Can you work these out from the model? Positions are in its coordinate system, mm. A direction names the side the tool comes from. Give positions to 0.01 mm unless a question says otherwise; leave off trailing zeros. Loops run counter-clockwise (first coordinate to the right, second up) from the corner with the lowest first, then second, coordinate; pieces in that order, holes last. Notation, with made-up numbers: (26, 58) - (71, 58) arc R18 ccw to (71, 93) - close; hole circle Ø9 at (-22, 18). An arc over 180 degrees is marked (long way). Answer as a JSON object with one key per item and string values.
```python
from build123d import *

# Parameters (mm, degrees)
F0_W     = 88.9
F0_H     = 88.9
F1_DEPTH = 2.54
F2_W     = 81.28
F2_H     = 81.28
F2_W_2   = 73.834833
F2_H_2   = 73.66
F3_DEPTH = 6.35
F4_R     = 1.27
F5_DEPTH = 2.541


with BuildPart() as f1:
    # F0 (on Top) → F1 (new body)
    with BuildSketch(Plane.XY):
        with Locations((44.45, 44.45)):
            Rectangle(F0_W, F0_H)
    extrude(amount=F1_DEPTH)

    # F2 (on face) → F3 (join)
    with BuildSketch(Plane.XY.offset(2.54)):
        with Locations((44.45, 44.45)):
            Rectangle(F2_W, F2_H)
        with Locations((44.362583, 44.45)):
            Rectangle(F2_W_2, F2_H_2, mode=Mode.SUBTRACT)
    extrude(amount=F3_DEPTH)

    # F4 (on face) → F5 (cut, through all)
    with BuildSketch(Plane.XY.offset(2.54)):
        with Locations((11.041525, 77.692158)):
            Circle(F4_R)
        with Locations((77.683642, 77.692158)):
            Circle(F4_R)
        with Locations((77.683642, 11.207842)):
            Circle(F4_R)
        with Locations((11.041525, 11.207842)):
            Circle(F4_R)
    extrude(amount=-F5_DEPTH, mode=Mode.SUBTRACT)


solid = f1.part
```
1) Imagine slicing it at B-B on y = 37. Write out the boundary of the cut face in (x, z), and give its area (3 significant figures).
Check sheet entries:
{"outline": "(0, 0) - (88.9, 0) - (88.9, 2.54) - (85.09, 2.54) - (85.09, 8.89) - (81.28, 8.89) - (81.28, 2.54) - (7.45, 2.54) - (7.45, 8.89) - (3.81, 8.89) - (3.81, 2.54) - (0, 2.54) - close", "area": "273 mm2"}
2) Which directions (+Z, -Z, +X, -X, +Y, -Y) give clear straight access to the entire face, cutting with the end or side of a thin tool? Please do faces 5 (the flat face through (44, 85.09, 6)), 6 (the flat face through (44, 81.28, 6)), 7 (the flat face through (3.81, 44, 6)).
Check sheet entries:
{"face 5": "+Z, +X, -X, +Y", "face 6": "+Z", "face 7": "+Z, -X, +Y, -Y"}
3) If we mould it in two halves opening along Y, with no side actions, what happens to faces 1 (the flat face through (44, 45, 2.54)), 2 (the flat face through (88.9, 44, 1)), 3 (the flat face through (44, 7.62, 6)), 4 (the flat face through (44, 88.9, 1))? For each: released by +Y, released by -Y, zero draft, split by the parting line, or undercut.
Check sheet entries:
{"face 1": "undercut", "face 2": "zero draft", "face 3": "undercut", "face 4": "released by +Y"}
4) Imagine slicing it at C-C on x = 80. Write out the boundary of the cut face in (y, z), and give its area (3 significant figures).
Check sheet entries:
{"outline": "(0, 0) - (88.9, 0) - (88.9, 2.54) - (85.09, 2.54) - (85.09, 8.89) - (81.28, 8.89) - (81.28, 2.54) - (7.62, 2.54) - (7.62, 8.89) - (3.81, 8.89) - (3.81, 2.54) - (0, 2.54) - close", "area": "274 mm2"}
5) I'm going to push flat-ended pins straight in: P1, Ø3, axis at x = 77.68, y = 11.21, coming from the +Z side; P2, Ø5, axis at x = 52, z = 6.5, coming from the +Y side; P3, Ø1.5, axis at y = 60, z = 7.5, coming from the +X side. Where does each tip first touch, or does it pass through?
Check sheet entries:
{"P1": "z = 2.54", "P2": "y = 85.09", "P3": "x = 85.09"}
6) I need wall thicknesses on L1, parallel to X at y = 66, z = 6.25; L2, parallel to Y at x = 8.5, z = 3.75; L3, parallel to Z at x = 8, y = 80. Which ranges of each line are inside material? Lowest first, please.
Check sheet entries:
{"L1": "3.81 to 7.45, 81.28 to 85.09", "L2": "3.81 to 7.62, 81.28 to 85.09", "L3": "0 to 2.54"}
7) Imagine slicing it at A-A on z = 4. Write out the boundary of the cut face in (x, y).
Check sheet entries:
{"outline": "(3.81, 3.81) - (85.09, 3.81) - (85.09, 85.09) - (3.81, 85.09) - close; hole (7.45, 7.62) - (81.28, 7.62) - (81.28, 81.28) - (7.45, 81.28) - close"}
